Model file for the job. Use its own axes, mm. Face numbers are marked on the shaded views. A direction names the side the tool comes from. Coordinates: 2 decimals unless noted, no trailing zeros. Order: outer loops, then holes, each group sorted by start corner. A loop starts at its lowest first (then second) coordinate and runs counter-clockwise, first axis right, second up. Notation, with made-up numbers: (4.5, -29.5) -> (42.5, -29.5) arc R30 cw to (42.5, 5.5) -> close; hole circle Ø10 at (-3, 34). An arc over 180 degrees is marked (long way). Use CSV: the item, a comma, the result in double quotes. Start each with the question number.
(1) Pull direction Y, two halves, no side cores. Call the marked faces 1, 2 and 3: pulls with the +Y half, pulls with the -Y half, needs draft (parallel to the pull), parting line crosses it, or undercut.
(2) Pin check, flat tips, straight feed: pin 1 Ø9 at (x, y) = (-43.307, 0) entering from -Z; pin 2 Ø10 at (x, z) = (37.5, 17.5) entering from -Y; pin 3 Ø2 at (y, z) = (7, 25) entering from -X; pin 4 Ø3.5 at (x, z) = (-32, 24.5) entering from +Y. Stop position of each tip, or through.
(3) Cut at D-D on y = 35. Write the cut outline in (x, z), plus the area to 3 significant figures.
(4) Cut at C-C on z = 13.75. Write the cut outline in (x, y), plus the area to 3 significant figures.
(5) Cut at A-A on y = 0. Write the cut outline in (x, z) (3 decimals), plus the area to 3 significant figures.
(6) Cut at B-B on x = 40. Write the cut outline in (y, z).
(7) Probe L1, parallel to Y at x = 0, z = 6.75 (3 decimals); L2, parallel to Y at x = 0, z = 24.25; L3, parallel to X at y = -1.5, z = 7.5. List the from-to ranges inside material, lowest first.
(8) Tool access for the marked faces 4, 5 and 6: list every direction of +Z, -Z, +X, -X, +Y, -Y with a clear straight run to the whole face (end or side of a thin tool).
```python
from build123d import *

# Parameters (mm, degrees)
SKETCH1_R          = 55.372
EXTRUDE1_DEPTH     = 29.464
SKETCH4_R          = 13.716
CUT_EXTRUDE1_DEPTH = 29.464
SKETCH5_R          = 19.558
CUT_EXTRUDE2_DEPTH = 11.176
SKETCH6_W          = 66.904134355
SKETCH6_H          = 50.8
CUT_REVOLVE1_ANGLE = 8
CUT_EXTRUDE4_START = 15.748
CUT_EXTRUDE4_DEPTH = 14.716
SKETCH12_R         = 5.588
CUT_EXTRUDE5_DEPTH = 30.464
CIRPATTERN1_COUNT  = 4


with BuildPart() as part:
    # Sketch1 → Extrude1 (new body)
    with BuildSketch(Plane.XY):
        Circle(SKETCH1_R)
    extrude(amount=EXTRUDE1_DEPTH)

    # Sketch4 → Cut-Extrude1 (cut)
    with BuildSketch(Plane.XY.offset(29.464)):
        Circle(SKETCH4_R)
    extrude(amount=-CUT_EXTRUDE1_DEPTH, mode=Mode.SUBTRACT)

    # Sketch5 → Cut-Extrude2 (cut)
    with BuildSketch(Plane.XY.offset(29.464)):
        Circle(SKETCH5_R)
    extrude(amount=-CUT_EXTRUDE2_DEPTH, mode=Mode.SUBTRACT)

    # Sketch6 → Cut-Revolve1 (revolve, cut)
    with BuildSketch(Plane.XY.offset(29.464)):
        with Locations((33.452067178, 0)):
            Rectangle(SKETCH6_W, SKETCH6_H)
    cut_revolve1 = revolve(axis=Axis((0, 25.4, 29.464), (0, 1, 0)), revolution_arc=CUT_REVOLVE1_ANGLE, mode=Mode.SUBTRACT)

    # Mirror1: Cut-Revolve1 across plane
    add(cut_revolve1.mirror(Plane(origin=(0, 0, 0), x_dir=(0, 0, 1), z_dir=(1, 0, 0))), mode=Mode.SUBTRACT)

    # Sketch9 → Cut-Extrude4 (cut, through all)
    with BuildSketch(Plane.XY.offset(CUT_EXTRUDE4_START)):
        with BuildLine():
            Line((-12.065, 43.307), (-12.065, 67.279112083))
            Line((-12.065, 67.279112083), (12.065, 66.235281078))
            Line((12.065, 66.235281078), (12.065, 43.307))
            ThreePointArc((12.065, 43.307), (0, 31.242), (-12.065, 43.307))
        make_face()
    cut_extrude4 = extrude(amount=CUT_EXTRUDE4_DEPTH, mode=Mode.SUBTRACT)

    # Sketch12 → Cut-Extrude5 (cut, through all)
    with BuildSketch(Plane.XY):
        with Locations((0, 43.307)):
            Circle(SKETCH12_R)
    cut_extrude5 = extrude(amount=CUT_EXTRUDE5_DEPTH, mode=Mode.SUBTRACT)

    # CirPattern1: Cut-Extrude4, Cut-Extrude5 ×4 about axis
    cirpattern1_axis = Axis((0, 0, 0), (0, 0, 1))
    for i in range(1, CIRPATTERN1_COUNT):
        add(cut_extrude4.rotate(cirpattern1_axis, i * 360 / CIRPATTERN1_COUNT), mode=Mode.SUBTRACT)
        add(cut_extrude5.rotate(cirpattern1_axis, i * 360 / CIRPATTERN1_COUNT), mode=Mode.SUBTRACT)


solid = part.part
```
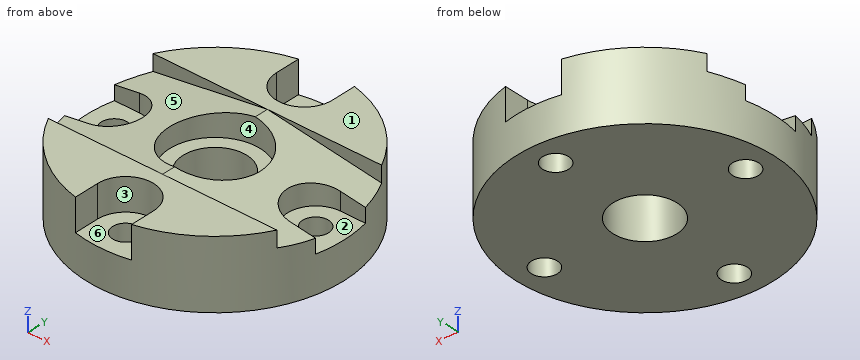
Outcome:
1,face 1,"needs draft"
1,face 2,"undercut"
1,face 3,"pulls with the -Y half"
2,pin 1,"through"
2,pin 2,"y = -44.83"
2,pin 3,"x = -34.22"
2,pin 4,"y = 46.38"
3,outline,"(-42.91, 0) -> (42.91, 0) -> (42.91, 29.46) -> (8.75, 29.46) -> (8.75, 15.75) -> (-8.75, 15.75) -> (-8.75, 29.46) -> (-42.91, 29.46) -> close"
3,area,"2,290 mm2"
4,outline,"circle Ø110.74 at (0, 0); hole circle Ø11.18 at (-43.31, 0); hole circle Ø27.43 at (0, 0); hole circle Ø11.18 at (0, -43.31); hole circle Ø11.18 at (0, 43.31); hole circle Ø11.18 at (43.31, 0)"
4,area,"8,650 mm2"
5,outline,"(-55.372, 0) -> (-48.895, 0) -> (-48.895, 15.748) -> (-55.372, 15.748) -> close; (-37.719, 0) -> (-13.716, 0) -> (-13.716, 18.288) -> (-19.558, 18.288) -> (-19.558, 26.715) -> (-31.242, 25.073) -> (-31.242, 15.748) -> (-37.719, 15.748) -> close; (13.716, 0) -> (37.719, 0) -> (37.719, 15.748) -> (31.242, 15.748) -> (31.242, 25.073) -> (19.558, 26.715) -> (19.558, 18.288) -> (13.716, 18.288) -> close; (48.895, 0) -> (55.372, 0) -> (55.372, 15.748) -> (48.895, 15.748) -> close"
5,area,"1,230 mm2"
6,outline,"(-38.29, 0) -> (-4.5, 0) -> (-4.5, 15.75) -> (-11.6, 15.75) -> (-11.6, 23.84) -> (-25.4, 23.84) -> (-25.4, 29.46) -> (-38.29, 29.46) -> close; (4.5, 0) -> (38.29, 0) -> (38.29, 29.46) -> (25.4, 29.46) -> (25.4, 23.84) -> (11.6, 23.84) -> (11.6, 15.75) -> (4.5, 15.75) -> close"
7,L1,"-55.372 to -48.895, -37.719 to -13.716, 13.716 to 37.719, 48.895 to 55.372"
7,L2,"-31.24 to -19.56, 19.56 to 31.24"
7,L3,"-55.35 to -48.69, -37.92 to -13.63, 13.63 to 37.92, 48.69 to 55.35"
8,face 4,"+Z"
8,face 5,"+Z, -X"
8,face 6,"+Z, -Y"
